Verification items for this drawing (mm, ordinates from the low corner). A direction names the side the tool comes from. Give positions to 0.01 mm unless a question says otherwise; leave off trailing zeros. Loops run counter-clockwise (first coordinate to the right, second up) from the corner with the lowest first, then second, coordinate; pieces in that order, holes last. Notation, with made-up numbers: (-18, -18.5) -> (2, -18.5) arc R15 ccw to (2, 4.5) -> close; hole circle Ø7 at (84.5, 89). An arc over 180 degrees is marked (long way). Write each question's results on one line, items separated by ' | '. Start each with the question number.
Item 1: Mould release check, pull along Z, two halves, no side actions. Record for the marked faces 1, 2 and 3: pulls with the +Z half, pulls with the -Z half, needs draft (parallel to the pull), parting line crosses it, or undercut.
Item 2: Cross-section at D-D on z = 34. Enter the section's corners in (x, y), then the cut area to 3 significant figures.
Item 3: Gauge pin test, flat ends, axial feed: pin 1 Ø1.5 at (y, z) = (2, 34) entering from -X; pin 2 Ø5.5 at (x, z) = (15, 34) entering from +Y; pin 3 Ø4.5 at (x, z) = (42.25, 4) entering from +Y. Record the tip position at first contact, or that the pin passes through.
Item 4: Cross-section at B-B on x = 42.25. Enter the section's corners in (y, z), then the cut area to 3 significant figures.
Item 5: Scan lines: line 1 along X through (y, z) = (2.1, 34); line 2 along Z through (x, y) = (15, 1.95); line 3 along X through (y, z) = (1.3, 4). Record each from-to range of solid material in increasing order.
Item 6: Cross-section at A-A on z = 4. Enter the section's corners in (x, y).
Item 7: Access from +Z, -Z, +X, -X, +Y, -Y to the whole of each face (thin tool, end or side, straight path). Record for the marked faces 4, 5 and 6.
Item 8: Cross-section at C-C on y = 2.55. Enter the section's corners in (x, z), then the cut area to 3 significant figures.
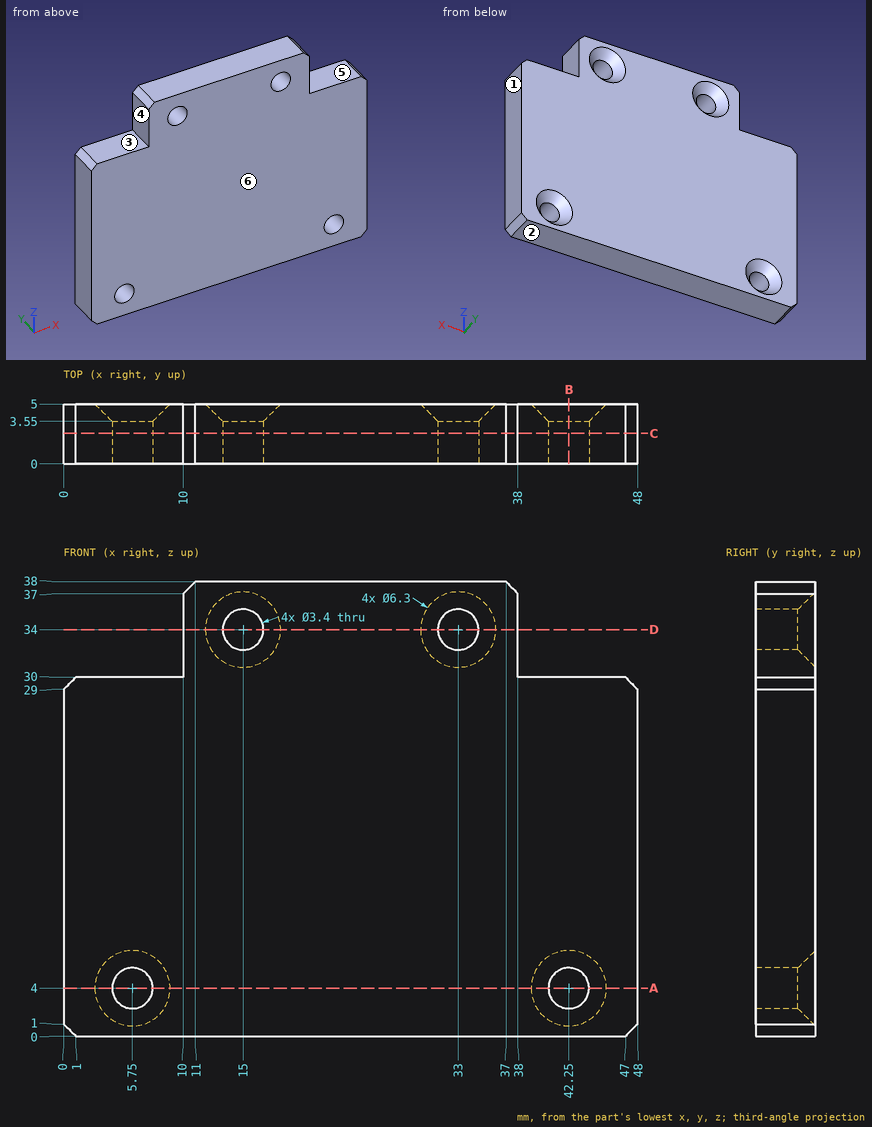
Answer sheet:
1) face 1: needs draft | face 2: pulls with the -Z half | face 3: pulls with the +Z half
2) outline: (10, 0) -> (13.3, 0) -> (13.3, 3.55) -> (11.85, 5) -> (10, 5) -> close; (16.7, 0) -> (31.3, 0) -> (31.3, 3.55) -> (29.85, 5) -> (18.15, 5) -> (16.7, 3.55) -> close; (34.7, 0) -> (38, 0) -> (38, 5) -> (36.15, 5) -> (34.7, 3.55) -> close | area: 102 mm²
3) pin 1: stops at x = 10 | pin 2: stops at y = 4.6 | pin 3: stops at y = 4.1
4) outline: (0, 0) -> (5, 0) -> (5, 0.85) -> (3.55, 2.3) -> (0, 2.3) -> close; (0, 5.7) -> (3.55, 5.7) -> (5, 7.15) -> (5, 30) -> (0, 30) -> close | area: 131 mm²
5) line 1: x = 10 to 13.3, 16.7 to 31.3, 34.7 to 38 | line 2: z = 0 to 32.3, 35.7 to 38 | line 3: x = 0 to 4.05, 7.45 to 40.55, 43.95 to 48
6) outline: (0, 0) -> (4.05, 0) -> (4.05, 3.55) -> (2.6, 5) -> (0, 5) -> close; (7.45, 0) -> (40.55, 0) -> (40.55, 3.55) -> (39.1, 5) -> (8.9, 5) -> (7.45, 3.55) -> close; (43.95, 0) -> (48, 0) -> (48, 5) -> (45.4, 5) -> (43.95, 3.55) -> close
7) face 4: +Z, -X, +Y, -Y | face 5: +Z, +X, +Y, -Y | face 6: +Z, -Z, +X, -X, -Y
8) outline: (0, 1) -> (1, 0) -> (47, 0) -> (48, 1) -> (48, 29) -> (47, 30) -> (38, 30) -> (38, 37) -> (37, 38) -> (11, 38) -> (10, 37) -> (10, 30) -> (1, 30) -> (0, 29) -> close; hole circle Ø3.4 at (5.75, 4); hole circle Ø3.4 at (15, 34); hole circle Ø3.4 at (33, 34); hole circle Ø3.4 at (42.25, 4) | area: 1,620 mm²
